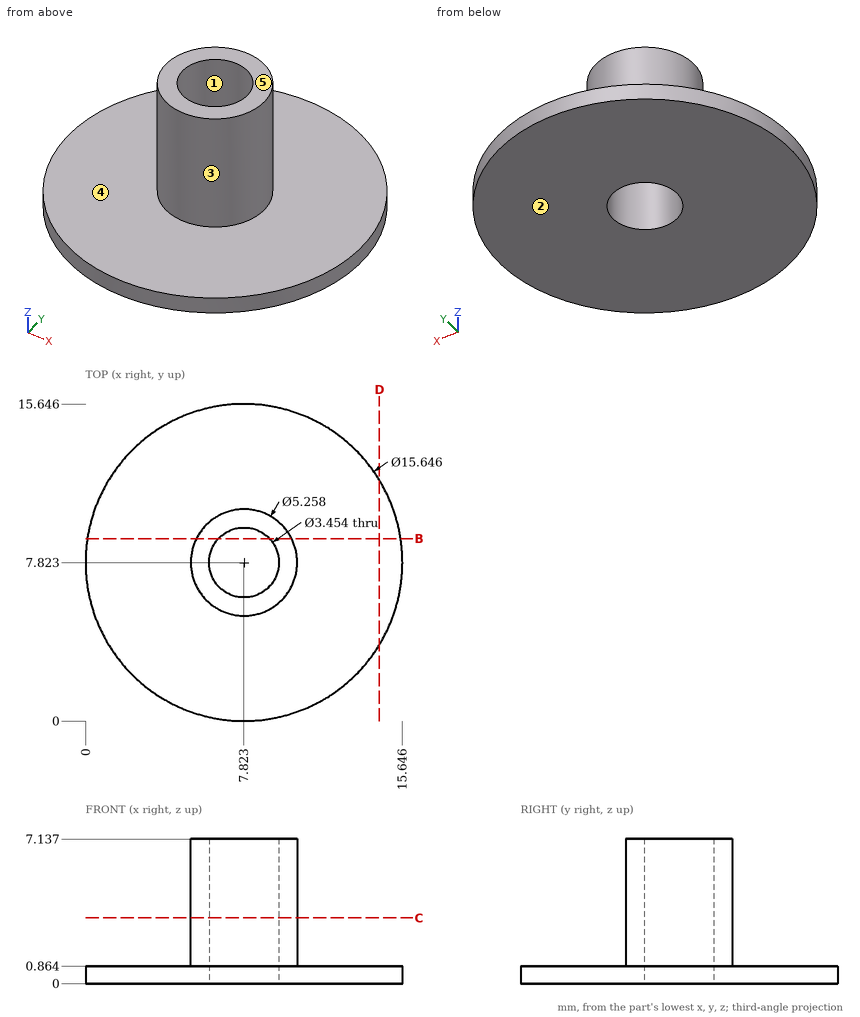
Geometry: see drawing. Coordinates: mm, zero at the bounding-box minimum. A direction names the side the tool comes from. Give positions to 0.01 mm unless a question says otherwise; leave off trailing zeros. Order: outer loops, then holes, each group sorted by start corner. A loop starts at its lowest first (then second) coordinate and runs counter-clockwise, first axis right, second up. Notation, with made-up numbers: M 10.25,15 L 31.25,15 A13 cw 31.25,22 Z; hole C -8,-2 d3. An arc over 180 degrees is marked long. Answer as CSV lines item,"result". Start each with the question number.
1) Mould query, pull axis X, two halves, no side actions, for the marked faces 1, 2 and 3. Classes: +X half, -X half, draft (parallel to the pull), parting line (faces both ways), or undercut.
2) Line query: line 1 (Z direction, x = 6.5, y = 4.25); line 2 (Y direction, x = 8.75, z = 3.5) (1 decimal); line 3 (Y direction, x = 9, z = 1.5) (1 decimal). Output: solid intervals per line, ascending. Write a range as from..to.
3) Cut plane C-C (z = 3.25). Output: boundary loops of the cut face in (x, y) (1 decimal).
4) Cut plane B-B (y = 9). Output: boundary loops of the cut face in (x, z).
5) First-contact query: P1, Ø1.5, axis at x = 6, z = 3, coming from the -Y side; P2, Ø1, axis at x = 8, z = 3.5, coming from the -Y side; P3, Ø1.5, axis at y = 9.5, z = 5, coming from the +X side. Flat tips, straight axial feed; report the tip coordinate or a pass-through.
6) Cut plane D-D (x = 14.5). Output: boundary loops of the cut face in (y, z).
7) Set-up query: the marked faces 4 and 5. Return all of +Z, -Z, +X, -X, +Y, -Y with unobstructed straight access to the full face (end or side cutting, diameter ignored); none if empty.
Findings below:
1,face 1,"undercut"
1,face 2,"draft"
1,face 3,"parting line"
2,line 1,"z = 0..0.86"
2,line 2,"y = 5.4..6.4, 9.3..10.3"
2,line 3,"y = 5.5..6.6, 9.1..10.2"
3,outline,"C 7.8,7.8 d5.3; hole C 7.8,7.8 d3.5"
4,outline,"M 0.09,0 L 6.56,0 L 6.56,7.14 L 5.47,7.14 L 5.47,0.86 L 0.09,0.86 Z; M 9.09,0 L 15.56,0 L 15.56,0.86 L 10.17,0.86 L 10.17,7.14 L 9.09,7.14 Z"
5,P1,"stops at y = 5.42"
5,P2,"stops at y = 5.19"
5,P3,"stops at x = 10.28"
6,outline,"M 3.75,0 L 11.9,0 L 11.9,0.86 L 3.75,0.86 Z"
7,face 4,"+Z"
7,face 5,"+Z, +X, -X, +Y, -Y"
